Input: part model. Units: mm. Frame: model coordinates. Coordinates: 2 decimals unless noted, no trailing zeros. Order: outer loops, then holes, each group sorted by start corner. A loop starts at its lowest first (then second) coordinate and runs counter-clockwise, first axis right, second up. Notation, with made-up numbers: (20, -4.5) - (31, -4.5) arc R18 cw to (31, 28.5) - close; hole circle Ø1 at (-26, 76.5). An arc over 180 degrees is marked (long way). One line per question, with ' | ' between items. Start each with the question number.
```python
from build123d import *

# Parameters (mm, degrees)
SKETCH1_W             = 300
SKETCH1_H             = 200
BOSS_EXTRUDE1_DEPTH   = 3
SKETCH2_W             = 145
SKETCH2_H             = 120
CUT_EXTRUDE1_DEPTH    = 3
SKETCH3_W             = 5
SKETCH3_H             = 160
CUT_EXTRUDE2_DEPTH    = 3
F_3_0MM_DOWEL_HOLE1_D = 3


with BuildPart() as part:
    # Sketch1 → Boss-Extrude1 (new body)
    with BuildSketch(Plane.XY):
        with Locations((150, 100)):
            Rectangle(SKETCH1_W, SKETCH1_H)
    extrude(amount=BOSS_EXTRUDE1_DEPTH)

    # Sketch2 → Cut-Extrude1 (cut)
    with BuildSketch(Plane.XY):
        with Locations((227.5, 100)):
            Rectangle(SKETCH2_W, SKETCH2_H)
    extrude(amount=CUT_EXTRUDE1_DEPTH, mode=Mode.SUBTRACT)

    # Sketch3 → Cut-Extrude2 (cut)
    with BuildSketch(Plane.XY):
        with Locations((27.5, 100)):
            Rectangle(SKETCH3_W, SKETCH3_H)
    extrude(amount=CUT_EXTRUDE2_DEPTH, mode=Mode.SUBTRACT)

    # Ø3.0mm Dowel Hole1 (through all)
    with Locations(Plane(origin=(0, 0, 0), x_dir=(-1, 0, 0), z_dir=(0, 0, -1))):
        with Locations((-85, 75), (-55, 75), (-55, 15), (-85, 15), (-295, 5), (-275, 25), (-85, 185), (-55, 185), (-55, 125), (-85, 125), (-275, 175), (-295, 195)):
            Hole(F_3_0MM_DOWEL_HOLE1_D / 2)


solid = part.part
```
(1) Pin query (flat end, axial travel): pin 1 (2.5 mm diameter, centred on x = 295, y = 195, fed in from -Z); pin 2 (0.9 mm diameter, centred on y = 104, z = 1, fed in from +X). Return the tip coordinate at first contact, or that it passes through.
(2) Material intervals for line 1 along Y through (x, z) = (85, 1.2); line 2 along Y through (x, z) = (275, 1.1); line 3 along X through (y, z) = (175, 0.95), sorted ascending. Write a range as from..to.
(3) Section B-B (y = 79.5). Output: boundary loops of the cut face in (x, z), then the cut area to 3 significant figures.
(4) Section C-C (x = 254.5). Output: boundary loops of the cut face in (y, z), then the cut area to 3 significant figures.
(5) Section A-A (z = 1.8). State how many separate pieces and enclosed holes the cut face has, then the cut area to 3 significant figures.
Worked answers:
1) pin 1: passes through | pin 2: stops at x = 155
2) line 1: y = 0..13.5, 16.5..73.5, 76.5..123.5, 126.5..183.5, 186.5..200 | line 2: y = 0..23.5, 26.5..40, 160..173.5, 176.5..200 | line 3: x = 0..25, 30..273.5, 276.5..300
3) outline: (0, 0) - (25, 0) - (25, 3) - (0, 3) - close; (30, 0) - (155, 0) - (155, 3) - (30, 3) - close | area: 450 mm²
4) outline: (0, 0) - (40, 0) - (40, 3) - (0, 3) - close; (160, 0) - (200, 0) - (200, 3) - (160, 3) - close | area: 240 mm²
5) separate pieces: 1 | enclosed holes: 13 | area: 41,700 mm²
